Source: CAD feature listing. Evaluate the final solid. Frame: model axes, mm. A direction names the side the tool comes from. Coordinates: 2 decimals unless noted, no trailing zeros. Answer as CSV lines item,"result".
Autodesk Inventor part; units mm, degrees
ref_plane "YZ Plane" through (0, 0, 0) normal (1, 0, 0) x (0, 1, 0)
ref_plane "XZ Plane" through (0, 0, 0) normal (0, 1, 0) x (-1, 0, 0)
ref_plane "XY Plane" through (0, 0, 0) normal (0, 0, 1) x (1, 0, 0)
sketch "Sketch1" plane through (0, 0, 0) normal (0, 0, 1) x (1, 0, 0)
  circle A0 centre (0, 0) radius 5
  circle A1 centre (0, 0) radius 34.5
  dimension "d0" = 10
  dimension "d1" = 69
extrude "Extrusion1" add sketch "Sketch1" along normal blind 5
sketch "Sketch2" plane through (0, 0, 5) normal (0, 0, 1) x (1, 0, 0)
  circle A0 centre (0, 0) radius 24.75
  circle A1 centre (0, 0) radius 34.5
  dimension "d4" = 49.5
extrude "Extrusion2" add sketch "Sketch2" along normal blind 14
sketch "Sketch3" plane through (0, 0, 5) normal (0, 0, 1) x (1, 0, 0)
  circle A0 centre (0, 0) radius 12.4
  circle A1 centre (0, 0) radius 5
  dimension "d7" = 24.8
extrude "Extrusion3" add sketch "Sketch3" along normal blind 20
chamfer "Chamfer1" distance 4 angle 15 1 edges at (-12.4, 0, 5) measured on face at (12.2394, -1.9891, 18.3333)
sketch "Sketch4" plane through (0, 0, 25) normal (0, 0, 1) x (1, 0, 0)
  circle A0 centre (9, 0) radius 1.5
  circle A1 centre (6.364, 6.364) radius 1.5
  circle A2 centre (0, 9) radius 1.5
  circle A3 centre (-6.364, 6.364) radius 1.5
  circle A4 centre (-9, 0) radius 1.5
  circle A5 centre (-6.364, -6.364) radius 1.5
  circle A6 centre (0, -9) radius 1.5
  circle A7 centre (6.364, -6.364) radius 1.5
  point P0 (0, 0)
  dimension "d13" = 3
  dimension "d14" = 9
  dimension "d17" = 360
extrude "Extrusion4" cut sketch "Sketch4" against normal through all
sketch "Sketch5" plane through (0, 0, 19) normal (0, 0, 1) x (1, 0, 0)
  circle A0 centre (29.5, 0) radius 2
  circle A1 centre (20.8597, 20.8597) radius 2
  circle A2 centre (0, 29.5) radius 2
  circle A3 centre (-20.8597, 20.8597) radius 2
  circle A4 centre (-29.5, 0) radius 2
  circle A5 centre (-20.8597, -20.8597) radius 2
  circle A6 centre (0, -29.5) radius 2
  circle A7 centre (20.8597, -20.8597) radius 2
  point P0 (0, 0)
  dimension "d21" = 4
  dimension "d22" = 29.5
  dimension "d25" = 360
extrude "Extrusion5" cut sketch "Sketch5" against normal through all
sketch "Sketch8" plane through (0, 0, 19) normal (0, 0, 1) x (1, 0, 0)
  circle A0 centre (29.5, 0) radius 2
  circle A1 centre (29.5, 0) radius 2
  line L0 (29.5, 4.3301) -> (33.25, 2.1651)
  line L1 (33.25, 2.1651) -> (33.25, -2.1651)
  line L2 (33.25, -2.1651) -> (29.5, -4.3301)
  line L3 (29.5, -4.3301) -> (25.75, -2.1651)
  line L4 (25.75, -2.1651) -> (25.75, 2.1651)
  line L5 (25.75, 2.1651) -> (29.5, 4.3301)
  line L6 (17.7978, 23.9215) -> (21.9804, 25.0422)
  line L7 (21.9804, 25.0422) -> (25.0422, 21.9804)
  line L8 (25.0422, 21.9804) -> (23.9215, 17.7978)
  line L9 (23.9215, 17.7978) -> (19.7389, 16.6771)
  line L10 (19.7389, 16.6771) -> (16.6771, 19.7389)
  line L11 (16.6771, 19.7389) -> (17.7978, 23.9215)
  line L12 (-4.3301, 29.5) -> (-2.1651, 33.25)
  line L13 (-2.1651, 33.25) -> (2.1651, 33.25)
  line L14 (2.1651, 33.25) -> (4.3301, 29.5)
  line L15 (4.3301, 29.5) -> (2.1651, 25.75)
  line L16 (2.1651, 25.75) -> (-2.1651, 25.75)
  line L17 (-2.1651, 25.75) -> (-4.3301, 29.5)
  line L18 (-23.9215, 17.7978) -> (-25.0422, 21.9804)
  line L19 (-25.0422, 21.9804) -> (-21.9804, 25.0422)
  line L20 (-21.9804, 25.0422) -> (-17.7978, 23.9215)
  line L21 (-17.7978, 23.9215) -> (-16.6771, 19.7389)
  line L22 (-16.6771, 19.7389) -> (-19.7389, 16.6771)
  line L23 (-19.7389, 16.6771) -> (-23.9215, 17.7978)
  line L24 (-29.5, -4.3301) -> (-33.25, -2.1651)
  line L25 (-33.25, -2.1651) -> (-33.25, 2.1651)
  line L26 (-33.25, 2.1651) -> (-29.5, 4.3301)
  line L27 (-29.5, 4.3301) -> (-25.75, 2.1651)
  line L28 (-25.75, 2.1651) -> (-25.75, -2.1651)
  line L29 (-25.75, -2.1651) -> (-29.5, -4.3301)
  line L30 (-17.7978, -23.9215) -> (-21.9804, -25.0422)
  line L31 (-21.9804, -25.0422) -> (-25.0422, -21.9804)
  line L32 (-25.0422, -21.9804) -> (-23.9215, -17.7978)
  line L33 (-23.9215, -17.7978) -> (-19.7389, -16.6771)
  line L34 (-19.7389, -16.6771) -> (-16.6771, -19.7389)
  line L35 (-16.6771, -19.7389) -> (-17.7978, -23.9215)
  line L36 (4.3301, -29.5) -> (2.1651, -33.25)
  line L37 (2.1651, -33.25) -> (-2.1651, -33.25)
  line L38 (-2.1651, -33.25) -> (-4.3301, -29.5)
  line L39 (-4.3301, -29.5) -> (-2.1651, -25.75)
  line L40 (-2.1651, -25.75) -> (2.1651, -25.75)
  line L41 (2.1651, -25.75) -> (4.3301, -29.5)
  line L42 (23.9215, -17.7978) -> (25.0422, -21.9804)
  line L43 (25.0422, -21.9804) -> (21.9804, -25.0422)
  line L44 (21.9804, -25.0422) -> (17.7978, -23.9215)
  line L45 (17.7978, -23.9215) -> (16.6771, -19.7389)
  line L46 (16.6771, -19.7389) -> (19.7389, -16.6771)
  line L47 (19.7389, -16.6771) -> (23.9215, -17.7978)
  point P0 (0, 0)
  point P1 (20.8597, 20.8597)
  point P2 (0, 29.5)
  point P3 (-20.8597, 20.8597)
  point P4 (-29.5, 0)
  point P5 (-20.8597, -20.8597)
  point P6 (0, -29.5)
  point P7 (20.8597, -20.8597)
  dimension "d32" = 7.5
  dimension "d35" = 360
extrude "Extrusion7" cut sketch "Sketch8" against normal blind 4 contours A0 | L0 L1 L2 L3 L4 L5 | L6 L7 L8 L9 L10 L11 | L12 L13 L14 L15 L16 L17 | L18 L19 L20 L21 L22 L23 | L24 L25 L26 L27 L28 L29 | L30 L31 L32 L33 L34 L35 | L36 L37 L38 L39 L40 L41 | L42 L43 L44 L45 L46 L47
properties part number "CS01" material "ABS Plastic"
(1) Cut plane A-A (z = 10). State how many separate pieces and enclosed holes the cut face has, then the cut area to 3 significant figures.
Computed values:
separate pieces,"2"
enclosed holes,"18"
area,"2,060 mm^2"
(2) Material intervals for L1, parallel to Y at x = 0, z = 19.5; L2, parallel to Y at x = 7, z = 22.25; L3, parallel to X at y = 9.5, z = 13, sorted ascending. Write a range as [from, to].
Computed values:
L1,"[-12.4, -10.5], [-7.5, -5], [5, 7.5], [10.5, 12.4]"
L2,"[-10.24, -7.72], [-5.01, 5.01], [7.72, 10.24]"
L3,"[-33.17, -22.85], [-7.97, -1.41], [1.41, 7.97], [22.85, 33.17]"
(3) Access query for faces 1 (the cylindrical face through (-0.325, 7.536, 12.675)), 2 (the flat face through (-24.474, 19.86, 17.028)). Directions: +Z, -Z, +X, -X, +Y, -Y. A direction counts if a zero-diameter tool reaches every point of the face in a straight line with its end or side. Return the directions, or none.
Computed values:
face 1,"+Z, -Z"
face 2,"+Z"
(4) Pin query (flat end, axial travel): pin 1 Ø5 at (x, y) = (-20.86, -20.86) entering from -Z; pin 2 Ø8 at (y, z) = (17.5, 6.5) entering from +X; pin 3 Ø6 at (y, z) = (-24, 11) entering from +X; pin 4 Ø2 at (x, y) = (31, 0.5) entering from +Z. Return the tip coordinate at first contact, or that it passes through.
Computed values:
pin 1,"z = 0"
pin 2,"x = 31.75"
pin 3,"x = 27.37"
pin 4,"z = 15"
